Source: three-view drawing plus pictorial views. Frame: mm from the lowest corner of the part. A direction names the side the tool comes from. Give positions to 0.01 mm unless a question says otherwise; leave off trailing zeros. Order: outer loops, then holes, each group sorted by start corner. A loop starts at its lowest first (then second) coordinate and runs counter-clockwise, first axis right, second up. Notation, with made-up numbers: (34, 29) - (73, 29) arc R16 cw to (73, 41) - close; hole circle Ø7 at (-23.75, -6.75). An arc over 180 degrees is marked (long way). Answer in a Markdown table with one row per item. Add a question column.
1. Access query for the marked faces 1, 2, 3 and 4. Directions: +Z, -Z, +X, -X, +Y, -Y. A direction counts if a zero-diameter tool reaches every point of the face in a straight line with its end or side. Return the directions, or none.
2. Contact query for flat-ended pins moving along their axis: pin 1 (5 mm diameter, centred on x = 25.5, z = 22, fed in from +Y); pin 2 (11 mm diameter, centred on x = 17, y = 26, fed in from +Z); pin 3 (3 mm diameter, centred on x = 5.5, y = 18.5, fed in from +Z); pin 4 (2.5 mm diameter, centred on y = 25, z = 17, fed in from -X). Output: stop coordinate, or through.
3. Section query C-C on x = 3.25. Return loops of the section in (y, z).
4. Section query B-B on z = 17.25. Return loops of the section in (x, y).
5. Section query D-D on x = 23. Return loops of the section in (y, z), and give its area (3 significant figures).
6. Section query A-A on y = 21.25. Return loops of the section in (x, z).
7. Ray query, line 1 (X direction, y = 17.5, z = 10.75); line 2 (Z direction, x = 4, y = 28.5); line 3 (Z direction, x = 18.5, y = 21.5). Return the intervals inside material, ascending. Write a range as [from, to].
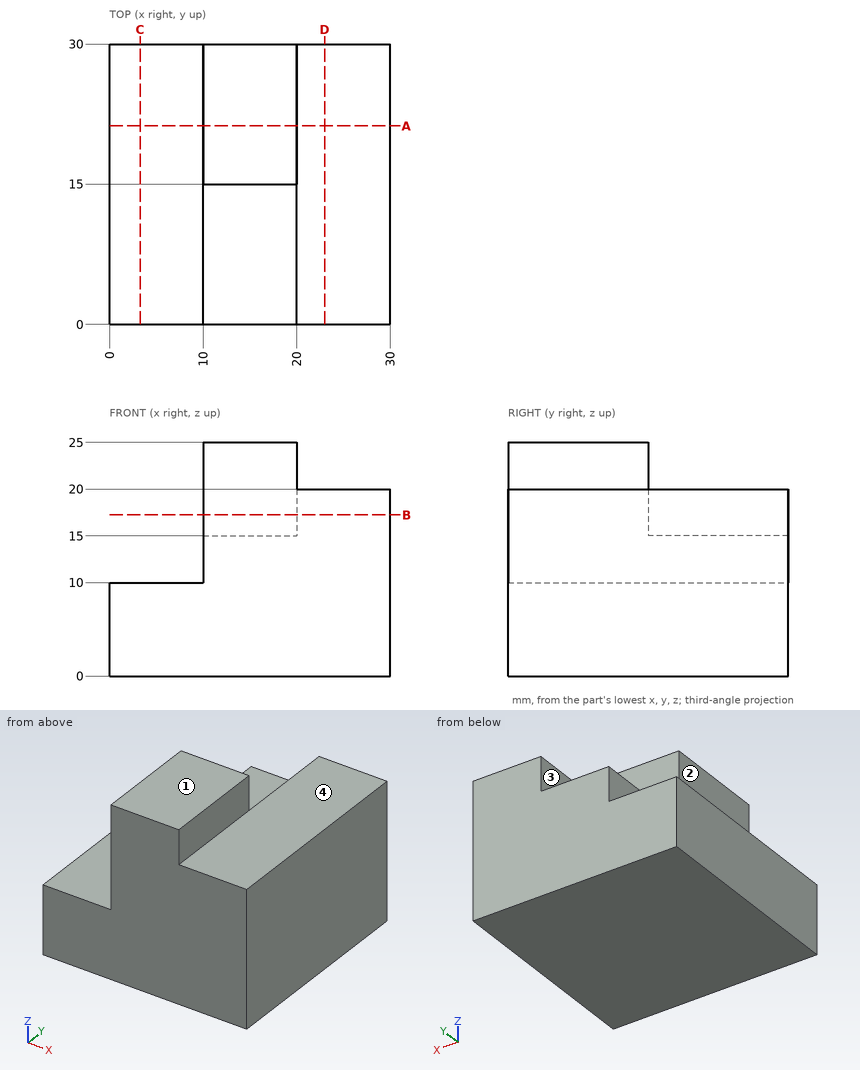
Answer:
| question | item | result |
|---|---|---|
| 1 | face 1 | +Z, +X, -X, +Y, -Y |
| 1 | face 2 | +Z, -X, +Y, -Y |
| 1 | face 3 | +Z, -X, +Y |
| 1 | face 4 | +Z, +X, +Y, -Y |
| 2 | pin 1 | stops at y = 30 |
| 2 | pin 2 | stops at z = 20 |
| 2 | pin 3 | stops at z = 10 |
| 2 | pin 4 | stops at x = 20 |
| 3 | outline | (0, 0) - (30, 0) - (30, 10) - (0, 10) - close |
| 4 | outline | (10, 0) - (30, 0) - (30, 30) - (20, 30) - (20, 15) - (10, 15) - close |
| 5 | outline | (0, 0) - (30, 0) - (30, 20) - (0, 20) - close |
| 5 | area | 600 mm² |
| 6 | outline | (0, 0) - (30, 0) - (30, 20) - (20, 20) - (20, 15) - (10, 15) - (10, 10) - (0, 10) - close |
| 7 | line 1 | x = [10, 30] |
| 7 | line 2 | z = [0, 10] |
| 7 | line 3 | z = [0, 15] |
